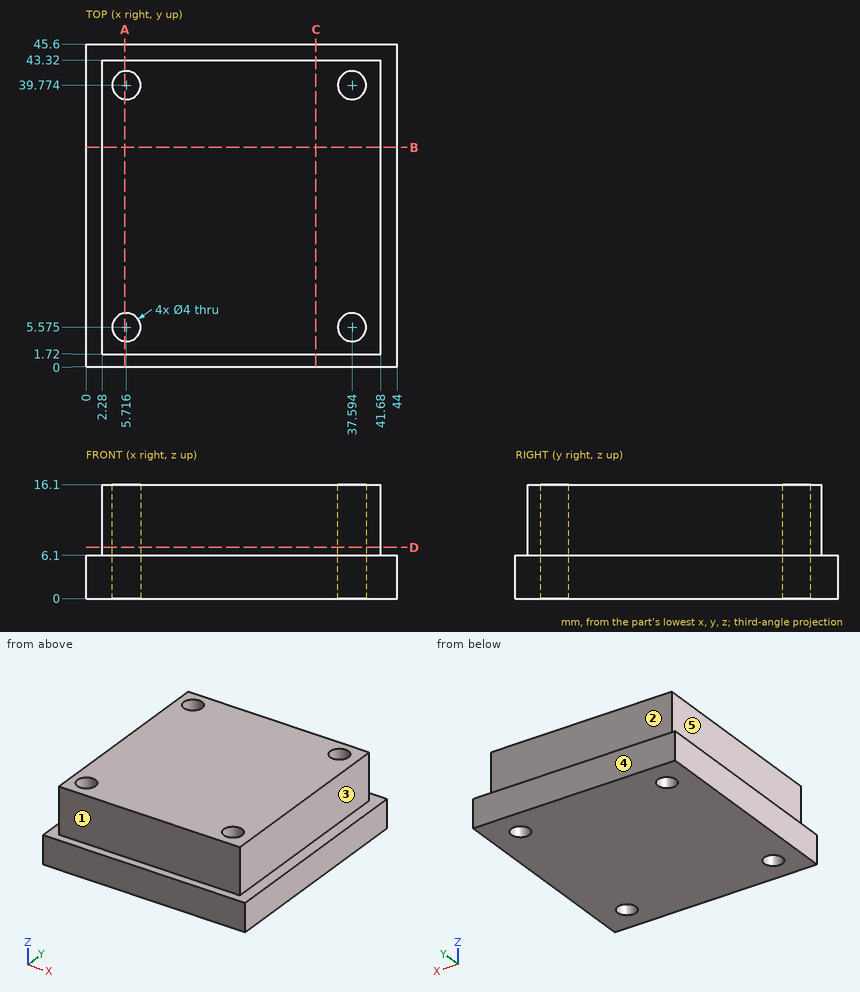
Design review of the part shown in the three views and the two pictorial views. Dimensions are in mm from the part's minimum x, y and z. A direction names the side the tool comes from. Coordinates: 2 decimals unless noted, no trailing zeros. Loops run counter-clockwise (first coordinate to the right, second up) from the corner with the lowest first, then second, coordinate; pieces in that order, holes last. Notation, with made-up numbers: M 17,16 L 37,16 A21 cw 37,43 Z; hole C -1.5,22 d2. An arc over 180 degrees is marked long. One line per question, with ' | ' between items.
(1) We need section B-B (y = 31). Give the boundary of the cut face in (x, z), and give its area (3 significant figures).
Filled in:
outline: M 0,0 L 44,0 L 44,6.1 L 41.68,6.1 L 41.68,16.1 L 2.28,16.1 L 2.28,6.1 L 0,6.1 Z | area: 662 mm^2
(2) We need section D-D (z = 7.25). Give the boundary of the cut face in (x, y) (1 decimal).
Filled in:
outline: M 2.3,1.7 L 41.7,1.7 L 41.7,43.3 L 2.3,43.3 Z; hole C 5.7,5.6 d4; hole C 5.7,39.8 d4; hole C 37.6,5.6 d4; hole C 37.6,39.8 d4
(3) We need section C-C (x = 32.5). Give the boundary of the cut face in (y, z).
Filled in:
outline: M 0,0 L 45.6,0 L 45.6,6.1 L 43.32,6.1 L 43.32,16.1 L 1.72,16.1 L 1.72,6.1 L 0,6.1 Z
(4) We need section A-A (x = 5.5). Give the boundary of the cut face in (y, z).
Filled in:
outline: M 0,0 L 3.59,0 L 3.59,16.1 L 1.72,16.1 L 1.72,6.1 L 0,6.1 Z; M 7.56,0 L 37.79,0 L 37.79,16.1 L 7.56,16.1 Z; M 41.76,0 L 45.6,0 L 45.6,6.1 L 43.32,6.1 L 43.32,16.1 L 41.76,16.1 Z
(5) Machinability: for the marked faces 1, 2, 3, 4 and 5, which of the approach directions +Z, -Z, +X, -X, +Y, -Y give a long, thin tool a straight path to every point of the face, cutting with its end or side? Answer none if there is none.
Filled in:
face 1: +Z, +X, -X, -Y | face 2: +Z, +X, -X, +Y | face 3: +Z, +X, +Y, -Y | face 4: +Z, -Z, +X, -X, +Y | face 5: +Z, -X, +Y, -Y
(6) Wall thickness on probe 1 along X at (y, z) = (40, 11.25); probe 2 along Y at (x, z) = (36, 6.25) (1 decimal); probe 3 along Y at (x, z) = (5, 1): over which ranges is each line inside the solid? List them lowest first.
Filled in:
probe 1: x = 2.28 to 3.73, 7.7 to 35.61, 39.58 to 41.68 | probe 2: y = 1.7 to 4.4, 6.8 to 38.6, 41 to 43.3 | probe 3: y = 0 to 3.71, 7.44 to 37.91, 41.64 to 45.6
(7) For pin 1 Ø3 at (y, z) = (20, 9.5) entering from +X, flat-tipped, find the tip position at first contact; note if it passes through.
Filled in:
pin 1: stops at x = 41.68
